The model under review builds one solid part; all positions refer to its coordinate system, in mm. Face numbers are marked on the shaded views. Round coordinates to 2 decimals unless told otherwise and drop trailing zeros. Write each loop counter-clockwise with the first axis right and the second up, starting at its lowest first coordinate (ties: lowest second). Pieces come first, ordered by that corner, then holes. Notation, with made-up numbers: (33.25, -12.75) - (39.25, -12.75) arc R15 cw to (39.25, 3.25) - close; hole circle Ø11 at (3.5, -32). An arc over 180 degrees is marked (long way). Use one line per item in the form item = value.
from build123d import *

# Parameters (mm, degrees)
BOSS_EXTRUDE1_START     = -2.5
BOSS_EXTRUDE1_OUTLINE_R = 31.45
BOSS_EXTRUDE1_DEPTH     = 5
SKETCH2_R               = 18.85
BOSS_EXTRUDE2_DEPTH     = 28.2
SKETCH3_R               = 19.15
BOSS_EXTRUDE3_DEPTH     = 5
SKETCH5_R               = 16
CUT_EXTRUDE2_DEPTH      = 59.629727954
FILLET7_R               = 2
CHAMFER2_SIZE           = 1
FILLET8_R               = 2.5
FILLET9_R               = 1.5


# Read off the part's stored shape, not the designer's step: Boss-Extrude1
with BuildPart() as part:
    # Boss-Extrude1 outline → Boss-Extrude1 (new body)
    with BuildSketch(Plane.XY.offset(BOSS_EXTRUDE1_START)):
        Circle(BOSS_EXTRUDE1_OUTLINE_R)
    extrude(amount=BOSS_EXTRUDE1_DEPTH)

    # Sketch2 → Boss-Extrude2 (add)
    with BuildSketch(Plane.XY.offset(2.5)):
        Circle(SKETCH2_R)
    extrude(amount=BOSS_EXTRUDE2_DEPTH)

    # Sketch3 → Boss-Extrude3 (add)
    with BuildSketch(Plane(origin=(0, 0, -2.5), x_dir=(-1, 0, 0), z_dir=(0, 0, -1))):
        with Locations(Location((0, 0, 0), (0, 0, 180))):
            Circle(SKETCH3_R)
    extrude(amount=BOSS_EXTRUDE3_DEPTH)

    # Sketch5 → Cut-Extrude2 (cut, through all)
    with BuildSketch(Plane.XY.offset(30.7)):
        Circle(SKETCH5_R)
    extrude(amount=-CUT_EXTRUDE2_DEPTH, mode=Mode.SUBTRACT)

    # Fillet7
    fillet7_edges = [part.edges().sort_by_distance(p)[0] for p in [
        (-18.85, 0, 2.5),
    ]]
    fillet(fillet7_edges, radius=FILLET7_R)

    # Chamfer2
    chamfer2_edges = [part.edges().sort_by_distance(p)[0] for p in [
        (-16, 0, 30.7),
    ]]
    chamfer(chamfer2_edges, length=CHAMFER2_SIZE)

    # Fillet8
    fillet8_edges = [part.edges().sort_by_distance(p)[0] for p in [
        (-31.45, 0, -2.5),
        (-31.45, 0, 2.5),
    ]]
    fillet(fillet8_edges, radius=FILLET8_R - 0.0001)  # a hair under: the kernel refuses the full size

    # Fillet9
    fillet9_edges = [part.edges().sort_by_distance(p)[0] for p in [
        (-19.15, 0, -7.5),
    ]]
    fillet(fillet9_edges, radius=FILLET9_R)


solid = part.part
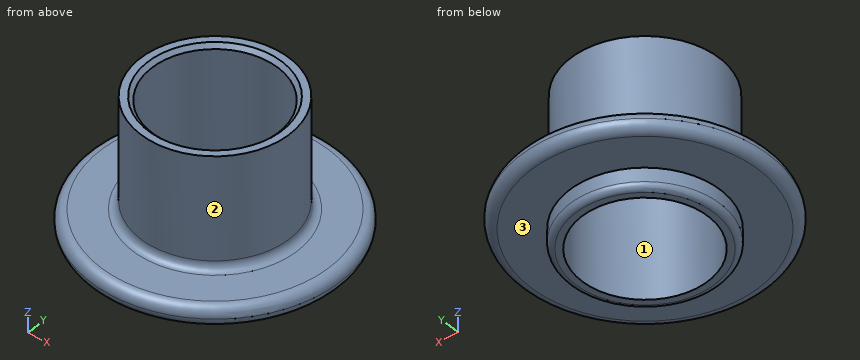
(1) Add section C-C on z = 6. Write out the cut boundary in (x, y), then the cut area to 3 significant figures.
Geometry results:
outline = circle Ø37.7 at (0, 0); hole circle Ø32 at (0, 0)
area = 312 mm2
(2) The part is to be moulded in two halves that separate along X. For the marked faces 1, 2 and 3, say which applies: +X half, -X half, draft (parallel to the pull), parting line (faces both ways), or undercut.
Geometry results:
face_1 = undercut
face_2 = parting line
face_3 = draft
(3) To check wall thickness, follow L1, parallel to Y at x = 0, z = 17; L2, parallel to X at y = -8, z = 20.5; L3, parallel to X at y = -1.5, z = -1. State the ranges of each line that lie inside material, in increasing order.
Geometry results:
L1 = -18.85 to -16, 16 to 18.85
L2 = -17.07 to -13.86, 13.86 to 17.07
L3 = -31.21 to -15.93, 15.93 to 31.21
(4) Insertion check: P1, Ø10, axis at y = 22.5, z = 17, coming from the -X side; P2, Ø8, axis at y = 19, z = 20, coming from the -X side; P3, Ø3, axis at x = 19, z = 15, coming from the -Y side; P4, Ø2, axis at x = 21, z = 17.5, coming from the +Y side. Each pin has a flat end and moves straight along its axis. Give the tip position at first contact, or say it passes through.
Geometry results:
P1 = -7.01
P2 = -11.42
P3 = -7.01
P4 = through
